The listing builds one solid part. Answer for the finished solid, in the listing's coordinates (mm). Face numbers are marked on the shaded views. Coordinates: 2 decimals unless noted, no trailing zeros. Loops run counter-clockwise (first coordinate to the right, second up) from the corner with the lowest first, then second, coordinate; pieces in that order, holes last. Notation, with made-up numbers: (60.25, 63) - (80.25, 63) arc R28 cw to (80.25, 85) - close; hole circle Ø10 at (-11, -9.5). An arc over 180 degrees is marked (long way). Return JSON: item names as keys, results as strings. Group by question number.
1. Find the intervals of material crossed by line 1 along Y through (x, z) = (0, 13.75); line 2 along Z through (x, y) = (10.5, -11) (3 decimals); line 3 along Y through (x, z) = (0, 3.5), in increasing order.
2. Section B-B (y = -65) is taken. Write down the section's boundary in (x, z) (3 decimals), and give its area (3 significant figures).
3. Section C-C (x = 10) is taken. Write down the section's boundary in (y, z) (3 decimals).
4. Section D-D (y = -90) is taken. Write down the section's boundary in (x, z), and give its area (3 significant figures).
5. Section A-A (z = 13.5) is taken. State how many separate pieces and enclosed holes the cut face has, and give its area (3 significant figures).
6. The mould has two halves that part along Y. Classify the marked faces 1, 2 and 3: pulls with the +Y half, pulls with the -Y half, needs draft (parallel to the pull), parting line crosses it, or undercut.
7. Each of these flat-tipped pins is pushed along its axis until it touches: P1, Ø10, axis at y = 69.5, z = 6.5, coming from the -X side; P2, Ø4.5, axis at x = -0.5, y = 90, coming from the +Z side; P3, Ø3, axis at y = 19.5, z = 5, coming from the +X side; P4, Ø1.5, axis at x = -18, z = 7.5, coming from the +Y side. Where does it stop, or does it pass through?
```python
from build123d import *

# Parameters (mm, degrees)
SKETCH2_W           = 40
SKETCH2_H           = 200
BOSS_EXTRUDE1_DEPTH = 20
SKETCH3_R           = 2
CUT_EXTRUDE1_DEPTH  = 10
FILLET1_R           = 20
SKETCH5_R           = 7.5
CUT_EXTRUDE3_DEPTH  = 10
FILLET2_R           = 18
SKETCH6_W           = 13.65
SKETCH6_H           = 150
CUT_EXTRUDE4_DEPTH  = 110.544511501
SKETCH7_W           = 5
SKETCH7_H           = 10
BOSS_EXTRUDE2_DEPTH = 15


with BuildPart() as part:
    # Sketch2 → Boss-Extrude1 (new body)
    with BuildSketch(Plane.XY):
        Rectangle(SKETCH2_W, SKETCH2_H)
    extrude(amount=BOSS_EXTRUDE1_DEPTH)

    # Sketch3 → Cut-Extrude1 (cut)
    with BuildSketch(Plane(origin=(0, 0, 0), x_dir=(-1, 0, 0), z_dir=(0, 0, -1))):
        with Locations((0, -90)):
            Circle(SKETCH3_R)
    extrude(amount=-CUT_EXTRUDE1_DEPTH, mode=Mode.SUBTRACT)

    # Fillet1
    fillet1_edges = [part.edges().sort_by_distance(p)[0] for p in [
        (20, -100, 10),
        (-20, -100, 10),
    ]]
    fillet(fillet1_edges, radius=FILLET1_R - 0.0001)  # a hair under: the kernel refuses the full size

    # Sketch5 → Cut-Extrude3 (cut)
    with BuildSketch(Plane.XY.offset(20)):
        with Locations((0, 88)):
            Circle(SKETCH5_R)
    extrude(amount=-CUT_EXTRUDE3_DEPTH, mode=Mode.SUBTRACT)

    # Fillet2
    fillet2_edges = [part.edges().sort_by_distance(p)[0] for p in [
        (-20, 100, 10),
        (20, 100, 10),
    ]]
    fillet(fillet2_edges, radius=FILLET2_R)

    # Sketch6 → Cut-Extrude4 (cut, through all)
    with BuildSketch(Plane.ZY.offset(20)):
        with Locations((10, -5)):
            Rectangle(SKETCH6_W, SKETCH6_H)
    extrude(amount=-CUT_EXTRUDE4_DEPTH, mode=Mode.SUBTRACT)

    # Sketch7 → Boss-Extrude2 (add)
    with BuildSketch(Plane(origin=(0, 0, 16.825), x_dir=(-1, 0, 0), z_dir=(0, 0, -1))):
        with Locations((17.5, -10)):
            Rectangle(SKETCH7_W, SKETCH7_H)
    boss_extrude2 = extrude(amount=BOSS_EXTRUDE2_DEPTH)

    # Mirror1: Boss-Extrude2 across plane
    add(boss_extrude2.mirror(Plane(origin=(0, 0, 0), x_dir=(0, 0, 1), z_dir=(1, 0, 0))))


solid = part.part
```
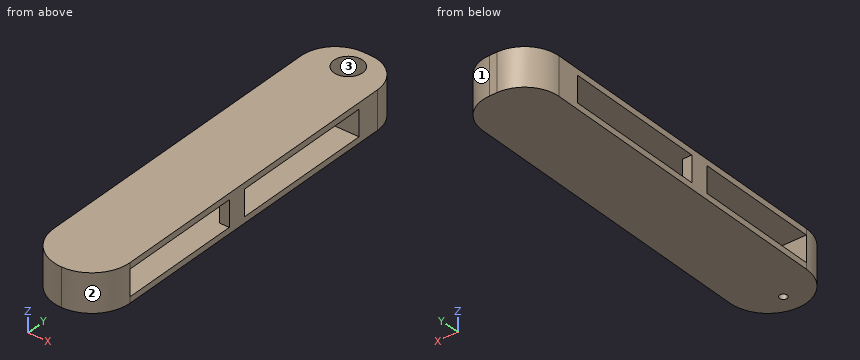
The answers:
{
 "1": {"line 1": "y = -100 to -80, 70 to 80.5, 95.5 to 100", "line 2": "z = 0 to 3.175, 16.825 to 20", "line 3": "y = -100 to -92, -88 to -80, 70 to 100"},
 "2": {"outline": "(-20, 0) - (20, 0) - (20, 3.175) - (-20, 3.175) - close; (-20, 16.825) - (20, 16.825) - (20, 20) - (-20, 20) - close", "area": "254 mm2"},
 "3": {"outline": "(-97.321, 0) - (98.125, 0) - (98.125, 20) - (-97.321, 20) - close; hole (-80, 3.175) - (70, 3.175) - (70, 16.825) - (-80, 16.825) - close"},
 "4": {"outline": "(-17.32, 0) - (-2, 0) - (-2, 10) - (2, 10) - (2, 0) - (17.32, 0) - (17.32, 20) - (-17.32, 20) - close", "area": "653 mm2"},
 "5": {"separate pieces": "4", "enclosed holes": "1", "area": "1,610 mm2"},
 "6": {"face 1": "pulls with the +Y half", "face 2": "pulls with the -Y half", "face 3": "undercut"},
 "7": {"P1": "stops at x = -20", "P2": "stops at z = 10", "P3": "passes through", "P4": "stops at y = 91.56"}
}
